Check sheet for the modelled part. Datum: model origin and axes. Units: mm. Face numbers are marked on the shaded views. Round coordinates to 2 decimals unless told otherwise and drop trailing zeros. Write each loop counter-clockwise with the first axis right and the second up, starting at its lowest first coordinate (ties: lowest second). Pieces come first, ordered by that corner, then holes.
Item 1: Section check C-C, the plane z = 20.5. Record the cut outline in (x, y), plus the area to 3 significant figures.
Item 2: Depth check by flat-ended pin: pin 1 (1 mm diameter, centred on x = -13, z = 50.5, fed in from -Y); pin 2 (1.1 mm diameter, centred on y = 37, z = 52.5, fed in from -X); pin 3 (1.9 mm diameter, centred on y = 37.5, z = 53, fed in from +X). Enter the tip coordinate at first touch or a pass-through.
Item 3: Release check for a two-part mould opening along Z. For the marked faces 1, 2 and 3 record: pulls with the +Z half, pulls with the -Z half, needs draft (parallel to the pull), parting line crosses it, or undercut.
Item 4: Material ranges on line 1 along Y through (x, z) = (-11, 55); line 2 along Y through (x, z) = (18, 14); line 3 along Z through (x, y) = (-21.5, -23), recorded low to high.
Item 5: Section check B-B, the plane y = 55. Record the cut outline in (x, z), plus the area to 3 significant figures.
Item 6: Section check A-A, the plane x = 0.5. Record the cut outline in (y, z), plus the area to 3 significant figures.
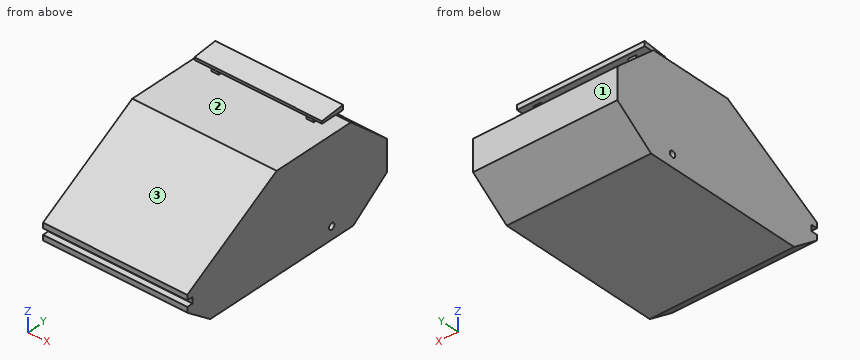
from build123d import *

# Parameters (mm, degrees)
F0_W      = 76.2
F0_H      = 127
F1_DEPTH  = 25.4
F2_W      = 76.2
F2_H      = 60.3884999398
F3_DEPTH  = 25.4
F5_DEPTH  = 25.4
F7_W      = 3.7973541766
F7_H      = 7.7133737504
F8_DEPTH  = 3.81
F9_W      = 67.4144178629
F9_H      = 12.7
F10_DEPTH = 2.54
F11_DEPTH = 25.4
F13_DEPTH = 119.38
F14_DEPTH = 157.988
F16_DEPTH = 160.7312
F18_DEPTH = 107.442
F19_DEPTH = 146.05
F22_DEPTH = 175.514
F23_R     = 1.6256
F24_DEPTH = 94.742
F25_W     = 85.8990699053
F25_H     = 3.175
F26_DEPTH = 3.175


with BuildPart() as f1:
    # F0 (on Top) → F1 (new body)
    with BuildSketch(Plane.XY):
        Rectangle(F0_W, F0_H)
    extrude(amount=F1_DEPTH)

    # F2 (on face) → F3 (join)
    with BuildSketch(Plane.XY.offset(25.4)):
        with Locations((0, -33.3057500301)):
            Rectangle(F2_W, F2_H)
    extrude(amount=F3_DEPTH)

    # F5 (add): a face of the model
    f5_faces = [f1.faces().sort_by_distance(p)[0] for p in [
        (0, 30.1942499699, 25.4),
    ]]
    extrude(f5_faces, amount=F5_DEPTH)

    # F7 (on face) → F8 (join)
    with BuildSketch(Plane.XY.offset(50.8)):
        with Locations((25.0877095386, 35.7790123671)):
            Rectangle(F7_W, F7_H)
        with Locations((-25.0877095386, 35.7790123671)):
            Rectangle(F7_W, F7_H)
    extrude(amount=F8_DEPTH)

    # F9 (on face) → F10 (join)
    with BuildSketch(Plane.XY.offset(54.61)):
        with Locations((0, 35.6483589858)):
            Rectangle(F9_W, F9_H)
    extrude(amount=F10_DEPTH)

    # F4 (on face) → F11 (join)
    with BuildSketch(Plane.YZ.offset(38.1)):
        Polygon((-63.5, 15.2083775029), (-3.1115000602, 50.8), (-63.5, 50.8), align=None)
    extrude(amount=F11_DEPTH)

    # F12 (on face) → F13 (cut)
    with BuildSketch(Plane.YZ.offset(63.5)):
        Polygon((-63.5, 50.8), (-63.5, 15.2083775029), (-3.1115000602, 50.8), align=None)
    extrude(amount=-F13_DEPTH, mode=Mode.SUBTRACT)

    # F6 (on face) → F14 (cut)
    with BuildSketch(Plane.YZ.offset(38.1)):
        Polygon((63.5, 50.8), (41.696511209, 50.8), (63.5, 31.4713791013), align=None)
    extrude(amount=-F14_DEPTH, mode=Mode.SUBTRACT)

    # F15 (on face) → F16 (cut)
    with BuildSketch(Plane.YZ.offset(33.7072089314)):
        Polygon((29.2983589858, 57.15), (29.2983589858, 55.88), (41.9983589858, 57.15), align=None)
    extrude(amount=-F16_DEPTH, mode=Mode.SUBTRACT)

    # F17 (on face) → F18 (cut)
    with BuildSketch(Plane.YZ.offset(38.1)):
        Polygon((-43.156321529, 0), (-63.5, 15.2083775029), (-63.5, 0), align=None)
    extrude(amount=-F18_DEPTH, mode=Mode.SUBTRACT)

    # F17 (on face) → F19 (cut)
    with BuildSketch(Plane.YZ.offset(38.1)):
        Polygon((63.5, 0), (63.5, 15.2083775029), (43.156321529, 0), align=None)
    extrude(amount=-F19_DEPTH, mode=Mode.SUBTRACT)

    # F21 (on face) → F22 (cut)
    with BuildSketch(Plane(origin=(-38.1, 0, 0), x_dir=(0, -1, 0), z_dir=(-1, 0, 0))):
        Polygon((67.4441531301, 13.2313063368), (56.999605149, 24.4063157588), (56.999605149, 6.1304802075), align=None)
    extrude(amount=-F22_DEPTH, mode=Mode.SUBTRACT)

    # F23 (on face) → F24 (cut)
    with BuildSketch(Plane.YZ.offset(38.1)):
        with Locations((30.1535148174, 6.5081091598)):
            Circle(F23_R)
    extrude(amount=-F24_DEPTH, mode=Mode.SUBTRACT)

    # F25 (on face) → F26 (cut)
    with BuildSketch(Plane.XZ.offset(56.999605149)):
        with Locations((0, 14.730398621)):
            Rectangle(F25_W, F25_H)
    extrude(amount=-F26_DEPTH, mode=Mode.SUBTRACT)


solid = f1.part
Values found:
1. outline: (-38.1, -54.52) - (38.1, -54.52) - (38.1, 63.5) - (-38.1, 63.5) - close
1. area: 8,990 mm2
2. pin 1: stops at y = -4.47
2. pin 2: stops at x = -26.99
2. pin 3: stops at x = 26.99
3. face 1: needs draft
3. face 2: undercut
3. face 3: pulls with the +Z half
4. line 1: y = 29.3 to 42
4. line 2: y = -53.82 to 61.88
4. line 3: z = 0 to 39.08
5. outline: (-38.1, 8.85) - (38.1, 8.85) - (38.1, 39.01) - (-38.1, 39.01) - close
5. area: 2,300 mm2
6. outline: (-57, 10.35) - (-43.16, 0) - (43.16, 0) - (63.5, 15.21) - (63.5, 31.47) - (41.7, 50.8) - (-3.11, 50.8) - (-57, 19.04) - (-57, 16.32) - (-53.82, 16.32) - (-53.82, 13.14) - (-57, 13.14) - close; (29.3, 54.61) - (42, 54.61) - (42, 57.15) - (29.3, 55.88) - close; hole circle Ø3.25 at (30.15, 6.51)
6. area: 4,830 mm2
